Can you work these out from the drawing? Everything is in mm from the part's minimum corner. A direction names the side the tool comes from. Coordinates: 2 decimals unless noted, no trailing zeros. Write each loop counter-clockwise with the first axis right and the second up, starting at its lowest first coordinate (ties: lowest second). Pieces come first, ordered by that corner, then holes. Notation, with made-up numbers: (58.5, -8) -> (74.5, -8) arc R26 cw to (74.5, 11) -> close; hole circle Ø2 at (77.5, 1.5). An arc over 180 degrees is marked (long way). Use CSV: the item, a comma, the result in double quotes. Start each with the question number.
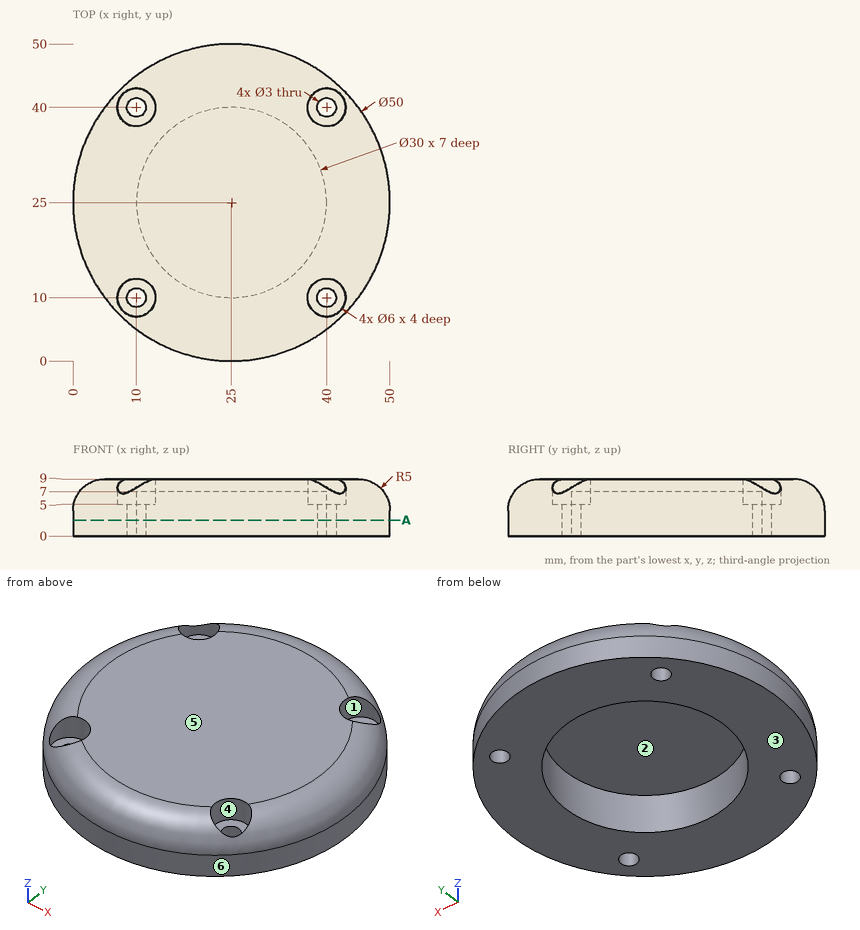
Item 1: I'm going to push flat-ended pins straight in: pin 1 (1.5 mm diameter, centred on y = 25.5, z = 4, fed in from -X); pin 2 (3.5 mm diameter, centred on x = 10, y = 40, fed in from +Z); pin 3 (1.8 mm diameter, centred on x = 40, y = 10, fed in from +Z); pin 4 (4 mm diameter, centred on y = 40.5, z = 4.5, fed in from -X). Where does each tip first touch, or does it pass through?
Item 2: Thinking about a two-plate mould opening in Y: for the marked faces 4, 5 and 6, which applies, +Y half, -Y half, draft (parallel to the pull), parting line (faces both ways), or undercut?
Item 3: Which directions (+Z, -Z, +X, -X, +Y, -Y) give clear straight access to the entire face, cutting with the end or side of a thin tool? Please do the marked faces 1, 2 and 3.
Item 4: I want a section at A-A on z = 2.5. Please give me the cut outline in (x, y), then the cut area to 3 significant figures.
Item 5: If I drill on line 1 along Y through (x, z) = (25, 3.5); line 2 along X through (y, z) = (24.5, 4) (3 decimals); line 3 along X through (y, z) = (39.5, 7.25), over which ranges is the centre line in solid material (lowest first)?
Geometry says:
1,pin 1,"x = 0"
1,pin 2,"z = 5"
1,pin 3,"through"
1,pin 4,"x = 3.98"
2,face 4,"undercut"
2,face 5,"draft"
2,face 6,"parting line"
3,face 1,"+Z"
3,face 2,"-Z"
3,face 3,"-Z, +X, -X, +Y, -Y"
4,outline,"circle Ø50 at (25, 25); hole circle Ø3 at (10, 10); hole circle Ø3 at (10, 40); hole circle Ø30 at (25, 25); hole circle Ø3 at (40, 10); hole circle Ø3 at (40, 40)"
4,area,"1,230 mm2"
5,line 1,"0 to 10, 40 to 50"
5,line 2,"0.005 to 10.008, 39.992 to 49.995"
5,line 3,"6.13 to 7.04, 12.96 to 37.04, 42.96 to 43.87"
